Geometry check sheet. Reference: drawing and pictorial views, mm from the part's lowest x, y, z. A direction names the side the tool comes from. Give positions to 0.01 mm unless a question says otherwise; leave off trailing zeros. Order: outer loops, then holes, each group sorted by start corner. A loop starts at its lowest first (then second) coordinate and runs counter-clockwise, first axis right, second up. Notation, with made-up numbers: (10.5, 35.25) - (31.5, 35.25) arc R5 cw to (31.5, 43.25) - close; hole circle Ø7 at (54, -30). An arc over 180 degrees is marked (long way). Answer as a JSON object with one key per item and string values.
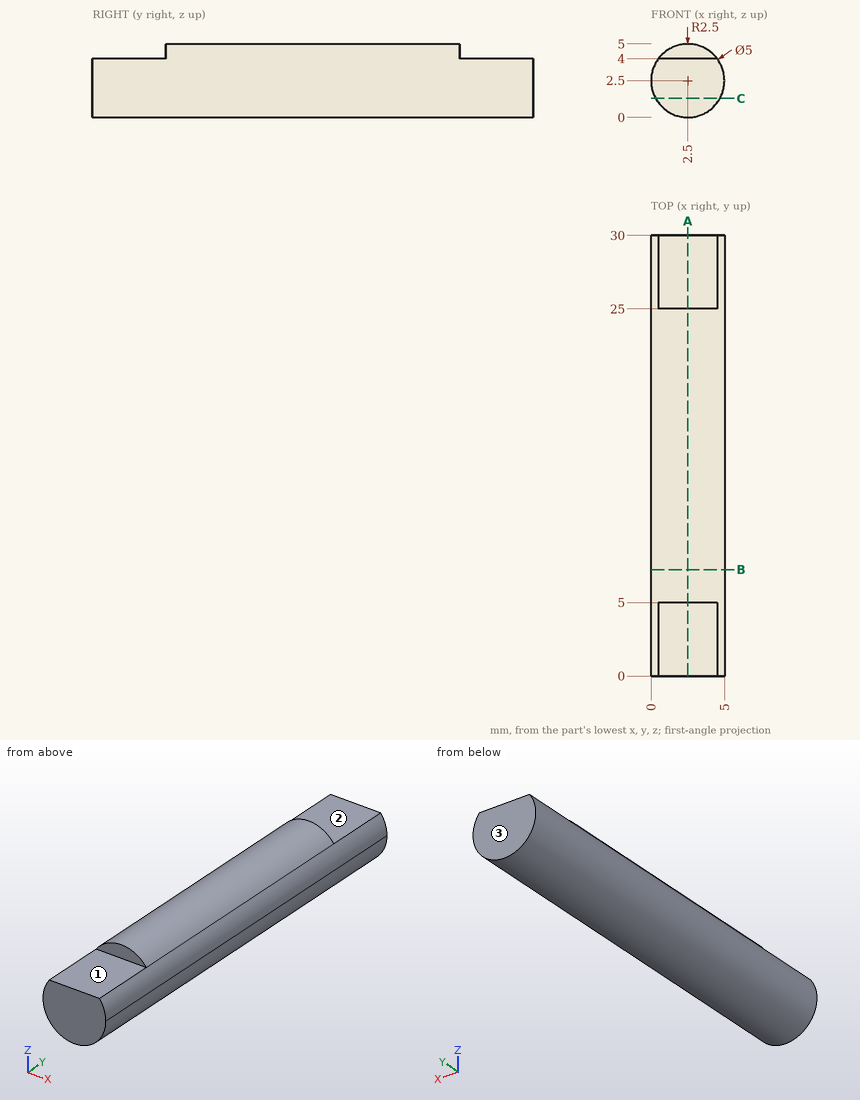
(1) Access from +Z, -Z, +X, -X, +Y, -Y to the whole of each face (thin tool, end or side, straight path). Record for the marked faces 1, 2 and 3.
Computed values:
{"face 1": "+Z, +X, -X, -Y", "face 2": "+Z, +X, -X, +Y", "face 3": "+Z, -Z, +X, -X, +Y"}
(2) Gauge pin test, flat ends, axial feed: pin 1 Ø1 at (y, z) = (21, 1.5) entering from +X; pin 2 Ø1 at (x, y) = (3.5, 20) entering from +Z; pin 3 Ø0.5 at (x, z) = (3.5, 4.5) entering from -Y. Record the tip position at first contact, or that the pin passes through.
Computed values:
{"pin 1": "stops at x = 4.95", "pin 2": "stops at z = 4.95", "pin 3": "stops at y = 5"}
(3) Material ranges on line 1 along Z through (x, y) = (2.65, 11); line 2 along Z through (x, y) = (3, 9.25); line 3 along X through (y, z) = (9, 4.25), recorded low to high. Write a range as [from, to].
Computed values:
{"line 1": "z = [0, 5]", "line 2": "z = [0.05, 4.95]", "line 3": "x = [0.71, 4.29]"}
(4) Section check B-B (y = 7.25). Record the cut outline in (x, z), then the cut area to 3 significant figures.
Computed values:
{"outline": "circle Ø5 at (2.5, 2.5)", "area": "19.6 mm²"}
(5) Section check C-C (z = 1.3). Record the cut outline in (x, y), then the cut area to 3 significant figures.
Computed values:
{"outline": "(0.31, 0) - (4.69, 0) - (4.69, 30) - (0.31, 30) - close", "area": "132 mm²"}
(6) Section check A-A (x = 2.5). Record the cut outline in (y, z).
Computed values:
{"outline": "(0, 0) - (30, 0) - (30, 4) - (25, 4) - (25, 5) - (5, 5) - (5, 4) - (0, 4) - close"}
